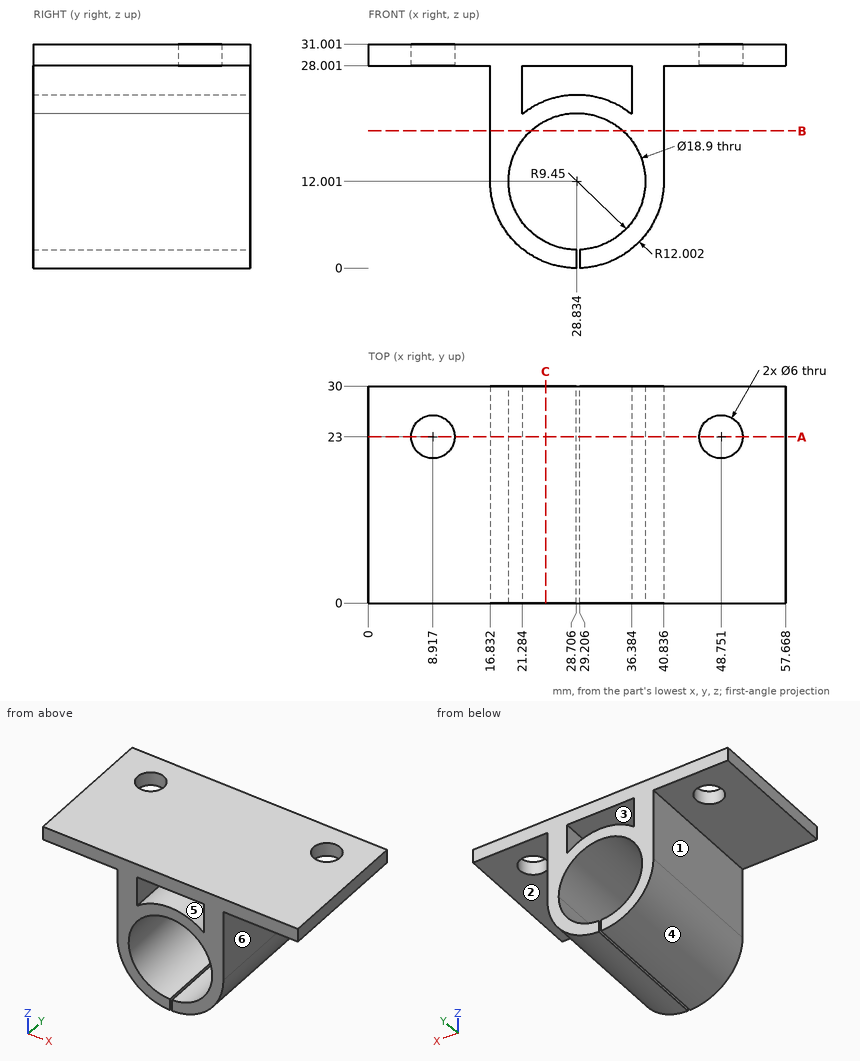
Study the drawing (mm; zero at the part's minimum x, y, z) and answer. A direction names the side the tool comes from. Coordinates: 2 decimals unless noted, no trailing zeros. Loops run counter-clockwise (first coordinate to the right, second up) from the corner with the lowest first, then second, coordinate; pieces in that order, holes last. Notation, with made-up numbers: M 50.25,35.5 L 94.25,35.5 A9 cw 94.25,49.5 Z; hole C 4,-13 d11. An arc over 180 degrees is marked long. Answer as a JSON object with one key per item and string values. Group by question number.
Item 1: Determine the mould class of the marked faces 4, 5 and 6 for opening direction Z: +Z half, -Z half, draft (parallel to the pull), parting line (faces both ways), or undercut.
Item 2: Section B-B (z = 19) is taken. Write down the section's boundary in (x, y).
Item 3: Consider L1, parallel to X at y = 11.5, z = 27; L2, parallel to Z at x = 25, y = 21.75 (1 decimal); L3, parallel to Z at x = 35.5, y = 27.25. Determine where each line is inside the solid, lowest interval first.
Item 4: Section A-A (y = 23) is taken. Give the number of separate pieces and of enclosed holes in the cut face, and give its area (3 significant figures).
Item 5: Section C-C (x = 24.5) is taken. Write down the section's boundary in (y, z), and give its area (3 significant figures).
Item 6: Each of these flat-tipped pins is pushed along its axis until it touches: P1, Ø3, axis at x = 8.5, y = 26, coming from the -Z side; P2, Ø10, axis at y = 25, z = 22.5, coming from the -X side; P3, Ø2, axis at y = 19, z = 1, coming from the -X side. Where does it stop, or does it pass through?
Item 7: Which of the six approach directions +Z, -Z, +X, -X, +Y, -Y give full straight-line access (tool end or side, diameter ignored) to the marked faces 1, 2 and 3?
Solved:
{
 "1": {"face 4": "-Z half", "face 5": "undercut", "face 6": "draft"},
 "2": {"outline": "M 16.83,0 L 22.48,0 L 22.48,30 L 16.83,30 Z; M 35.18,0 L 40.84,0 L 40.84,30 L 35.18,30 Z"},
 "3": {"L1": "x = 16.83 to 21.28, 36.38 to 40.84", "L2": "z = 0.6 to 3.4, 20.6 to 23.4, 28 to 31", "L3": "z = 2.02 to 5.3, 18.7 to 21.98, 28 to 31"},
 "4": {"separate pieces": "3", "enclosed holes": "1", "area": "392 mm2"},
 "5": {"outline": "M 0,0.81 L 30,0.81 L 30,3.6 L 0,3.6 Z; M 0,20.4 L 30,20.4 L 30,23.19 L 0,23.19 Z; M 0,28 L 30,28 L 30,31 L 0,31 Z", "area": "258 mm2"},
 "6": {"P1": "stops at z = 28", "P2": "stops at x = 16.83", "P3": "stops at x = 22.2"},
 "7": {"face 1": "-Z, -X, +Y, -Y", "face 2": "-Z, +X, +Y, -Y", "face 3": "+Y, -Y"}
}
